from build123d import *

# Parameters (mm, degrees)
CYLINDER007_R             = 9.5
CYLINDER007_DEPTH         = 2
FILLET007_R               = 0.5
CYLINDER006_R             = 9.5
CYLINDER006_DEPTH         = 2
FILLET006_R               = 0.5
FUSION005_PLACEMENT_ANGLE = 180


with BuildPart() as fillet007:
    # Cylinder007 → Cylinder007 (new body)
    with BuildSketch(Plane.XY.offset(12)):
        Circle(CYLINDER007_R)
    extrude(amount=CYLINDER007_DEPTH)

    # Fillet007
    fillet007_edges = [fillet007.edges().sort_by_distance(p)[0] for p in [
        (-9.5, 0, 14),
    ]]
    fillet(fillet007_edges, radius=FILLET007_R)


with BuildPart() as disc003:
    # Cylinder006 → Cylinder006 (new body)
    with BuildSketch(Plane.XY.offset(11)):
        Circle(CYLINDER006_R)
    extrude(amount=CYLINDER006_DEPTH)

    # Fillet006
    fillet006_edges = [disc003.edges().sort_by_distance(p)[0] for p in [
        (-9.5, 0, 11),
    ]]
    fillet(fillet006_edges, radius=FILLET006_R)


with BuildPart() as disc003_1:
    # Fillet006 placement: moved
    add(disc003.part.moved(Location((0, 0, -1))))

    # Fusion005: union Fillet007
    add(fillet007.part)


with BuildPart() as disc003_2:
    # Fusion005 placement: moved
    add(disc003_1.part.moved(Location((-17, -17, 24))).rotate(Axis((-17, -17, 24), (0, 1, 0)), FUSION005_PLACEMENT_ANGLE))


solid = disc003_2.part
Could you check a few things on this model? Use its own coordinates, in mm. Give positions to 0.01 mm unless a question says otherwise; leave off trailing zeros. Order: outer loops, then holes, each group sorted by start corner. A loop starts at its lowest first (then second) coordinate and runs counter-clockwise, first axis right, second up. Notation, with made-up numbers: (74.5, 71.5) - (95.5, 71.5) arc R20 cw to (95.5, 94.5) - close; hole circle Ø2 at (-36, 72). An arc over 180 degrees is marked (long way). One line per item, written item: value. Start each with the question number.
1. For P1, Ø1, axis at y = -18.5, z = 11, coming from the -X side, with a flat end and sliding along its axis, tell me the tip position at first contact or that it passes through.
2. If I drill on probe 1 along Y at (x, z) = (-16.5, 12.85); probe 2 along X at (y, z) = (-12.75, 10.3); probe 3 along Y at (x, z) = (-9.75, 12.3), over which ranges is the centre line in solid material (lowest first)?
3. Imagine slicing it at A-A on z = 12.5. List the corners of the cut face in (x, y) for me.
Values:
1. P1: x = -26.45
2. probe 1: -26.49 to -7.51
2. probe 2: -25.45 to -8.55
2. probe 3: -23.14 to -10.86
3. outline: circle Ø19 at (-17, -17)
